Design review of the part built by this model. Coordinates are the model's own, in mm. A direction names the side the tool comes from. Round coordinates to 2 decimals unless told otherwise and drop trailing zeros. Order: outer loops, then holes, each group sorted by start corner. A loop starts at its lowest first (then second) coordinate and runs counter-clockwise, first axis right, second up. Notation, with made-up numbers: (-39.5, 11.5) - (-3.5, 11.5) arc R19 cw to (-3.5, 27.5) - close; hole circle Ø1 at (15, 1.5). An arc over 180 degrees is marked (long way). Use CSV: the item, a comma, the result in double quotes.
from build123d import *

# Parameters (mm, degrees)
F2_R     = 5
F3_R     = 4.25
F4_DEPTH = 70


with BuildPart() as f1:
    # F0 (on Front) → F1 (revolve)
    with BuildSketch(Plane.XZ):
        with BuildLine():
            Line((-0.7845937077, 51.5), (-9.7845937077, 51.5))
            Line((-9.7845937077, 51.5), (-9.7845937077, 3.6967689234))
            Line((-9.7845937077, 3.6967689234), (-36.5961492169, -18.8007974156))
            Line((-36.5961492169, -18.8007974156), (-22.5946347751, -18.8007974156))
            Line((-22.5946347751, -18.8007974156), (-2.5706556593, -1.9986839248))
            ThreePointArc((-2.5706556593, -1.9986839248), (-1.2530547725, -0.2815530179), (-0.7845937077, 1.8315382908))
            Line((-0.7845937077, 1.8315382908), (-0.7845937077, 51.5))
        make_face()
    revolve(axis=Axis((-0.7845937077, 0, 26.6657691454), (0, 0, -1)))

    # F2
    f2_edges = [f1.edges().sort_by_distance(p)[0] for p in [
        (35.026962, 0, -18.800797),
    ]]
    fillet(f2_edges, radius=F2_R)

    # F3 (on face) → F4 (cut)
    with BuildSketch(Plane.XY.offset(51.5)):
        with Locations((-0.7845937077, 0)):
            Circle(F3_R)
    extrude(amount=-F4_DEPTH, mode=Mode.SUBTRACT)

    # F5 (on Front) → F6 (revolve, cut)
    with BuildSketch(Plane.XZ):
        Polygon((7.4, 51.5), (-0.8, 51.5), (-0.8, 35.5), (3.7, 35.5), align=None)
    revolve(axis=Axis((-0.8, 0, 43.5), (0, 0, -1)), mode=Mode.SUBTRACT)


solid = f1.part
1) We need section A-A (y = 0). Give the boundary of the cut face in (x, z), then the cut area to 3 significant figures.
Data:
outline,"(-26.07, -9.97) arc R5 ccw to (-22.86, -18.8) - (-22.59, -18.8) - (-5.03, -4.07) - (-5.03, 35.5) - (-5.3, 35.5) - (-9, 51.5) - (-9.78, 51.5) - (-9.78, 3.7) - close; (3.47, -4.07) - (21.03, -18.8) - (21.29, -18.8) arc R5 ccw to (24.5, -9.97) - (8.22, 3.7) - (8.22, 51.5) - (7.4, 51.5) - (3.7, 35.5) - (3.47, 35.5) - close"
area,"869 mm2"
2) For faces 4 (the face through (0.387, 8.923, 27.264)), 5 (the face through (3.27, 1.28, 15.99)), list the 3-axis set-ups (+Z, -Z, +X, -X, +Y, -Y) from which the entire face can be reached by the end or side of a thin tool; tool diameter is ignored.
Data:
face 4,"+Z"
face 5,"+Z, -Z"
3) The part is to be moulded in two halves that separate along X. For faces 1 (the face through (7, -6, 3)), 2 (the face through (0.32, -4.98, -4.78)), 3 (the face through (7, -4, 51.5)), say which applies: +X half, -X half, draft (parallel to the pull), parting line (faces both ways), or undercut.
Data:
face 1,"parting line"
face 2,"undercut"
face 3,"draft"
4) We need section C-C (z = 40.5). Give the boundary of the cut face in (x, y).
Data:
outline,"circle Ø18 at (-0.78, 0); hole circle Ø11.31 at (-0.8, 0)"
5) Insertion check: pin 1 Ø10 at (y, z) = (12, 27) entering from +X; pin 2 Ø3 at (y, z) = (-6.5, -3.5) entering from +X; pin 3 Ø12 at (y, z) = (4, 38.5) entering from -X; pin 4 Ø3 at (y, z) = (-11, 20.5) entering from -X. Each pin has a flat end and moves straight along its axis. Give the tip position at first contact, or say it passes through.
Data:
pin 1,"stops at x = 4.87"
pin 2,"stops at x = 17.53"
pin 3,"stops at x = -9.78"
pin 4,"passes through"
6) We need section B-B (z = 16). Give the boundary of the cut face in (x, y), then the cut area to 3 significant figures.
Data:
outline,"circle Ø18 at (-0.78, 0); hole circle Ø8.5 at (-0.78, 0)"
area,"198 mm2"
7) To check wall thickness, follow L1, parallel to Y at x = 4, z = -12.5; L2, parallel to Y at x = 8.5, z = -13; L3, parallel to Z at x = 18.5, y = 11.5. State the ranges of each line that lie inside material, in increasing order. Write a range as from..to.
Data:
L1,"y = -26.47..-13.48, 13.48..26.47"
L2,"y = -25.36..-11.65, 11.65..25.36"
L3,"z = -18.79..-7.59"
